Geometry: see drawing. Coordinates: mm, zero at the bounding-box minimum. A direction names the side the tool comes from. Round coordinates to 2 decimals unless told otherwise and drop trailing zeros. Order: outer loops, then holes, each group sorted by start corner. A loop starts at its lowest first (then second) coordinate and runs counter-clockwise, first axis right, second up. Notation, with made-up numbers: (10.5, -25) -> (27.5, -25) arc R17 ccw to (27.5, -11) -> close; hole circle Ø2 at (33.25, 49). An arc over 180 degrees is marked (long way). Write item = value, one per line. Start each with the question number.
(1) Draft query along Y for the marked faces 1, 2 and 3. Return one class per face: released by +Y, released by -Y, zero draft, split by the parting line, or undercut.
(2) Ray query, line 1 (Y direction, x = 8, z = 76) (1 decimal); line 2 (X direction, y = 104.5, z = 74.5); line 3 (X direction, y = 52.5, z = 69.5). Return the intervals inside material, ascending.
(3) Cut plane A-A on y = 179.5. Return the cut outline in (x, z).
(4) Reachability of the marked faces 4 and 5 from +Z, -Z, +X, -X, +Y, -Y: full face, straight path, thin tool, end or side. Return the list, or none.
(5) Cut plane B-B on z = 12. Return the cut outline in (x, y) (1 decimal).
(6) Cut plane C-C on x = 18. Return the cut outline in (y, z) (1 decimal).
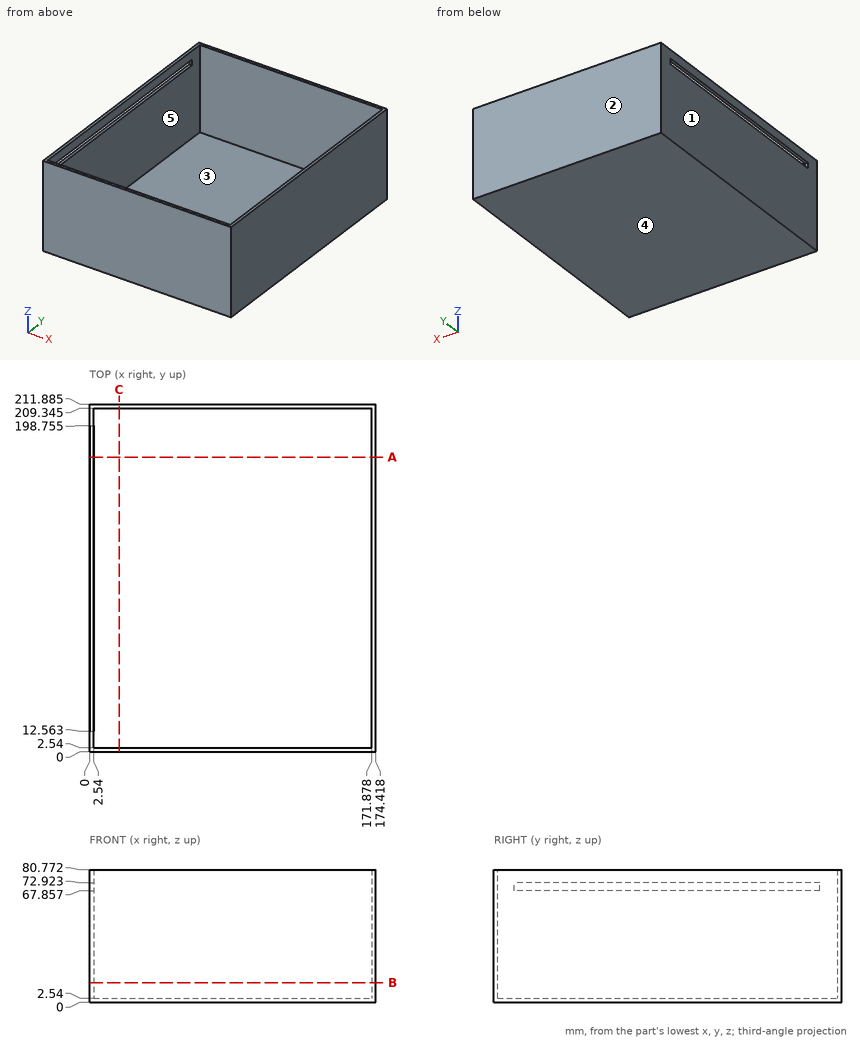
Evaluation:
q1.face_1 = zero draft
q1.face_2 = released by +Y
q1.face_3 = undercut
q2.line_1 = 0 to 2.5, 209.3 to 211.9
q2.line_2 = 0 to 2.54, 171.88 to 174.42
q2.line_3 = 171.88 to 174.42
q3.outline = (0, 0) -> (174.42, 0) -> (174.42, 80.77) -> (171.88, 80.77) -> (171.88, 2.54) -> (2.54, 2.54) -> (2.54, 67.86) -> (0, 67.86) -> close; (0, 72.92) -> (2.54, 72.92) -> (2.54, 80.77) -> (0, 80.77) -> close
q4.face_4 = -Z, +X, -X, +Y, -Y
q4.face_5 = +Z
q5.outline = (0, 0) -> (174.4, 0) -> (174.4, 211.9) -> (0, 211.9) -> close; hole (2.5, 2.5) -> (171.9, 2.5) -> (171.9, 209.3) -> (2.5, 209.3) -> close
q6.outline = (0, 0) -> (211.9, 0) -> (211.9, 80.8) -> (209.3, 80.8) -> (209.3, 2.5) -> (2.5, 2.5) -> (2.5, 80.8) -> (0, 80.8) -> close
